Geometry check sheet. Reference: the model listing, model coordinates, mm. Face numbers are marked on the shaded views. A direction names the side the tool comes from. Give positions to 0.01 mm unless a question says otherwise; leave off trailing zeros. Loops run counter-clockwise (first coordinate to the right, second up) from the corner with the lowest first, then second, coordinate; pieces in that order, holes last.
1. Release check for a two-part mould opening along X. For the marked faces 4, 5 and 6 record: +X half, -X half, draft (parallel to the pull), parting line (faces both ways), or undercut.
2. Cross-section at B-B, the plane y = 7.5. Record the cut outline in (x, z).
3. Cross-section at D-D, the plane y = 13.25. Record the cut outline in (x, z).
4. Material ranges on L1, parallel to X at y = 13.4, z = 37; L2, parallel to Z at x = 1.4, y = 7.5; L3, parallel to X at y = 1.75, z = 24, recorded low to high.
5. Go/stop test with flat-tipped pins: pin 1 Ø2 at (x, y) = (12.5, 1) entering from -Z; pin 2 Ø1.8 at (x, z) = (19, 37) entering from -Y. Record where each tip stops, or that it passes through.
6. Cross-section at C-C, the plane x = 19. Record the cut outline in (y, z), plus the area to 3 significant figures.
7. Cross-section at A-A, the plane z = 8. Record the cut outline in (x, y).
8. Tool access check on the marked faces 1, 2 and 3. Record the directions out of +Z, -Z, +X, -X, +Y, -Y that give a thin tool (end or side, any length) a straight path to the whole face; none if there is none.
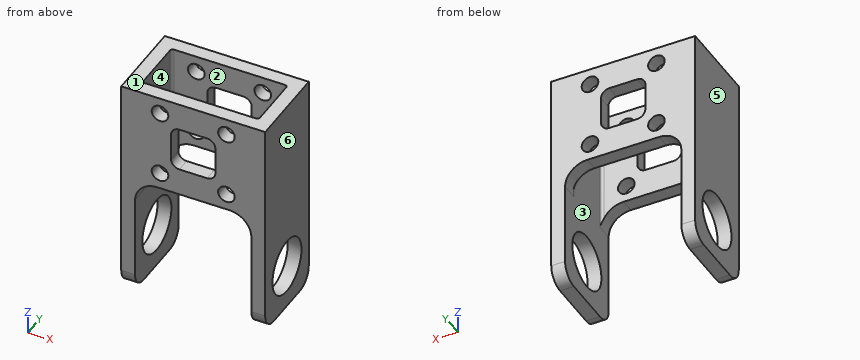
from build123d import *

# Parameters (mm, degrees)
SKETCH_1_W               = 23
SKETCH_1_H               = 15
EXTRUDE_1_DEPTH          = 40
SKETCH_2_W               = 20
SKETCH_2_H               = 10
CUT_EXTRUDE_2_DEPTH      = 68
SKETCH_5_W               = 20
SKETCH_5_H               = 22
CUT_EXTRUDE_5_DEPTH      = 20
SKETCH_6_R               = 5
CUT_EXTRUDE_6_DEPTH      = 20
SKETCH_7_R               = 1.5
CUT_EXTRUDE_7_DEPTH      = 20
SKETCH_8_W               = 3
SKETCH_8_H               = 15
EXTRUDE_2_DEPTH          = 40
SKETCH_9_W               = 21
SKETCH_9_H               = 10
CUT_EXTRUDE_8_DEPTH      = 100
CUT_EXTRUDE_9_DEPTH      = 20.5
CUT_EXTRUDE_9_DEPTH_BACK = 0.5
SKETCH_10_W              = 22
SKETCH_10_H              = 2.5
FILLET_4_R               = 0.5
CUT_EXTRUDE_START        = -4.5
SKETCH_11_R              = 5
CUT_EXTRUDE_10_DEPTH     = 4.5
FILLET_5_R               = 4
FILLET_6_R               = 3


with BuildPart() as part:
    # 草图1 → 凸台-拉伸1 (new body)
    with BuildSketch(Plane.XY):
        with Locations((11.5, 7.5)):
            Rectangle(SKETCH_1_W, SKETCH_1_H)
    extrude(amount=EXTRUDE_1_DEPTH)

    # 草图2 → 切除-拉伸2 (cut)
    with BuildSketch(Plane.XY.offset(40)):
        with Locations((13, 7.5)):
            Rectangle(SKETCH_2_W, SKETCH_2_H)
    extrude(amount=-CUT_EXTRUDE_2_DEPTH, mode=Mode.SUBTRACT)

    # 草图5 → 切除-拉伸5 (cut)
    with BuildSketch(Plane.XZ):
        with Locations((13, 11)):
            Rectangle(SKETCH_5_W, SKETCH_5_H)
    extrude(amount=-CUT_EXTRUDE_5_DEPTH, mode=Mode.SUBTRACT)

    # 草图6 → 切除-拉伸6 (cut)
    with BuildSketch(Plane(origin=(3, 0, 0), x_dir=(0, 0, -1), z_dir=(1, 0, 0))):
        with Locations(Location((-8, 7.5, 0), (0, 0, 90))):
            Circle(SKETCH_6_R)
    extrude(amount=-CUT_EXTRUDE_6_DEPTH, mode=Mode.SUBTRACT)

    # 草图7 → 切除-拉伸7 (cut)
    with BuildSketch(Plane.XZ):
        with Locations(Location((7, 37, 0), (0, 0, 270))):
            Circle(SKETCH_7_R)
        with Locations(Location((19, 37, 0), (0, 0, 270))):
            Circle(SKETCH_7_R)
        with Locations(Location((7, 25, 0), (0, 0, 270))):
            Circle(SKETCH_7_R)
        with Locations(Location((19, 25, 0), (0, 0, 270))):
            Circle(SKETCH_7_R)
        with BuildLine():
            Line((10.5, 27), (15.5, 27))
            ThreePointArc((15.5, 27), (16.560660172, 27.439339828), (17, 28.5))
            Line((17, 28.5), (17, 33.5))
            ThreePointArc((17, 33.5), (16.560660172, 34.560660172), (15.5, 35))
            Line((15.5, 35), (10.5, 35))
            ThreePointArc((10.5, 35), (9.439339828, 34.560660172), (9, 33.5))
            Line((9, 33.5), (9, 28.5))
            ThreePointArc((9, 28.5), (9.439339828, 27.439339828), (10.5, 27))
        make_face()
    extrude(amount=-CUT_EXTRUDE_7_DEPTH, mode=Mode.SUBTRACT)

    # 草图8 → 凸台-拉伸2 (add)
    with BuildSketch(Plane.XY.offset(40)):
        with Locations((24.5, 7.5)):
            Rectangle(SKETCH_8_W, SKETCH_8_H)
    extrude(amount=-EXTRUDE_2_DEPTH)

    # 草图9 → 切除-拉伸8 (cut)
    with BuildSketch(Plane.XY.offset(40)):
        with Locations((13, 7.5)):
            Rectangle(SKETCH_9_W, SKETCH_9_H)
    extrude(amount=-CUT_EXTRUDE_8_DEPTH, mode=Mode.SUBTRACT)

    # 草图10 → 切除-拉伸9 (cut, two sides: drawn at the far end of the back side and taken through both)
    with BuildSketch(Plane.ZY.offset(-23).offset(-CUT_EXTRUDE_9_DEPTH_BACK)):
        with Locations((11, 13.75)):
            Rectangle(SKETCH_10_W, SKETCH_10_H)
        with Locations((11, 1.25)):
            Rectangle(SKETCH_10_W, SKETCH_10_H)
    extrude(amount=CUT_EXTRUDE_9_DEPTH + CUT_EXTRUDE_9_DEPTH_BACK, mode=Mode.SUBTRACT)

    # 圆角4
    fillet_4_edges = [part.edges().sort_by_distance(p)[0] for p in [
        (2.5, 12.5, 31),
        (2.5, 2.5, 31),
        (23.5, 2.5, 31),
        (23.5, 12.5, 31),
    ]]
    fillet(fillet_4_edges, radius=FILLET_4_R)

    # 草图11 → 切除-拉伸10 (cut)
    with BuildSketch(Plane.ZY.offset(-23.5).offset(CUT_EXTRUDE_START)):
        with Locations(Location((8, 7.5, 0), (0, 0, 180))):
            Circle(SKETCH_11_R)
    extrude(amount=CUT_EXTRUDE_10_DEPTH, mode=Mode.SUBTRACT)

    # 圆角5
    fillet_5_edges = [part.edges().sort_by_distance(p)[0] for p in [
        (23.5, 13.5, 22),
        (23.5, 1.5, 22),
        (2.5, 13.5, 22),
        (2.5, 1.5, 22),
    ]]
    fillet(fillet_5_edges, radius=FILLET_5_R)

    # 圆角6
    fillet_6_edges = [part.edges().sort_by_distance(p)[0] for p in [
        (24.75, 15, 0),
        (24.75, 0, 0),
        (1.25, 15, 0),
        (1.25, 0, 0),
    ]]
    fillet(fillet_6_edges, radius=FILLET_6_R)


solid = part.part
Result:
1. face 4: undercut
1. face 5: -X half
1. face 6: +X half
2. outline: (0, 0) - (2.5, 0) - (2.5, 3) - (0, 3) - close; (0, 13) - (2.5, 13) - (2.5, 40) - (0, 40) - close; (23.5, 0) - (26, 0) - (26, 3) - (23.5, 3) - close; (23.5, 13) - (26, 13) - (26, 40) - (23.5, 40) - close
3. outline: (0, 0.27) - (2.5, 0.27) - (2.5, 18) arc R4 cw to (6.5, 22) - (19.5, 22) arc R4 cw to (23.5, 18) - (23.5, 0.27) - (26, 0.27) - (26, 40) - (0, 40) - close; hole circle Ø3 at (7, 25); hole circle Ø3 at (7, 37); hole (9, 28.5) arc R1.5 ccw to (10.5, 27) - (15.5, 27) arc R1.5 ccw to (17, 28.5) - (17, 33.5) arc R1.5 ccw to (15.5, 35) - (10.5, 35) arc R1.5 ccw to (9, 33.5) - close; hole circle Ø3 at (19, 25); hole circle Ø3 at (19, 37)
4. L1: x = 0 to 5.5, 8.5 to 17.5, 20.5 to 26
4. L2: z = 0 to 3, 13 to 40
4. L3: x = 0 to 5.88, 8.12 to 17.88, 20.12 to 26
5. pin 1: stops at z = 22
5. pin 2: passes through
6. outline: (0, 22) - (2.5, 22) - (2.5, 23.5) - (0, 23.5) - close; (0, 26.5) - (2.5, 26.5) - (2.5, 35.5) - (0, 35.5) - close; (0, 38.5) - (2.5, 38.5) - (2.5, 40) - (0, 40) - close; (12.5, 22) - (15, 22) - (15, 23.5) - (12.5, 23.5) - close; (12.5, 26.5) - (15, 26.5) - (15, 35.5) - (12.5, 35.5) - close; (12.5, 38.5) - (15, 38.5) - (15, 40) - (12.5, 40) - close
6. area: 60.0 mm2
7. outline: (0, 0) - (2.5, 0) - (2.5, 2.5) - (0, 2.5) - close; (0, 12.5) - (2.5, 12.5) - (2.5, 15) - (0, 15) - close; (23.5, 0) - (26, 0) - (26, 2.5) - (23.5, 2.5) - close; (23.5, 12.5) - (26, 12.5) - (26, 15) - (23.5, 15) - close
8. face 1: +Z, +X, -X, +Y, -Y
8. face 2: +Z, -Z
8. face 3: -Z
